Build history of the part. All positions in model axes, mm. Face numbers are marked on the shaded views. A direction names the side the tool comes from. Coordinates: 2 decimals unless noted, no trailing zeros. Order: outer loops, then holes, each group sorted by start corner. A loop starts at its lowest first (then second) coordinate and runs counter-clockwise, first axis right, second up. Notation, with made-up numbers: (84, 47) - (104, 47) arc R10 cw to (104, 60) - close; hole circle Ø4 at (65, 23.25). An arc over 180 degrees is marked (long way). Return JSON: item names as keys, results as strings.
Autodesk Inventor part; units mm, degrees
ref_plane "Work Plane1" through (0, 0, 24) normal (0, 0, 1) x (1, 0, 0)
ref_plane "YZ Plane" through (0, 0, 0) normal (1, 0, 0) x (0, 1, 0)
ref_plane "XZ Plane" through (0, 0, 0) normal (0, 1, 0) x (-1, 0, 0)
sketch "Sketch1" plane through (0, 0, 0) normal (0, 0, 1) x (1, 0, 0)
  line L0 (-9.7719, -3.7131) -> (-29.115, -3.7131)
  line L1 (-29.115, -3.7131) -> (-29.115, -8.7131)
  line L2 (-29.115, -8.7131) -> (-9.115, -8.7131)
  line L3 (-9.115, -8.7131) -> (-9.115, -28.7131)
  line L4 (-9.115, -28.7131) -> (-4.115, -28.7131)
  line L5 (-4.115, -28.7131) -> (-4.115, -9.37)
  line L6 (-9.7719, -3.7131) -> (27.9352, 33.994)
  line L7 (33.5921, 28.3372) -> (-4.115, -9.37)
  circle A0 centre (32.885, 33.2869) radius 1.85
  arc A1 (33.5921, 28.3372) -> (27.9352, 33.994) centre (32.885, 33.2869) ccw
  dimension "d0" = 20
  dimension "d1" = 20
  dimension "d2" = 5
  dimension "d3" = 5
  dimension "d7" = 42
  dimension "d8" = 42
  dimension "d9" = 3.7
  dimension "d18" = 5
  dimension "d19" = 135
  dimension "d67" = 8
extrude "Extrusion1" add sketch "Sketch1" along normal blind 30
ref_plane "Work Plane1" through (0, 0, 24) normal (0, 0, 1) x (1, 0, 0)
sketch "Sketch3" plane through (0, 0, 24) normal (0, 0, 1) x (1, 0, 0)
  circle A0 centre (32.885, 33.2869) radius 1.85
  circle A1 centre (32.885, 33.2869) radius 12.5
  point P0 (0, 0)
  dimension "d13" = 25
extrude "Extrusion3" cut sketch "Sketch3" against normal blind 18
sketch "Sketch5" plane through (0, 0, 0) normal (0, 0, -1) x (-1, 0, 0)
  circle A0 centre (-32.885, 33.2869) radius 1.85
  line L0 (29.115, -8.7131) -> (29.115, -3.7131)
  line L1 (29.115, -3.7131) -> (9.7719, -3.7131)
  line L2 (9.7719, -3.7131) -> (-27.9352, 33.994)
  arc A1 (-27.9352, 33.994) -> (-33.5921, 28.3372) centre (-32.885, 33.2869) ccw
  line L3 (-33.5921, 28.3372) -> (4.115, -9.37)
  line L4 (4.115, -9.37) -> (4.115, -28.7131)
  line L5 (4.115, -28.7131) -> (9.115, -28.7131)
  line L6 (9.115, -28.7131) -> (9.115, -8.7131)
  line L7 (9.115, -8.7131) -> (29.115, -8.7131)
  line L8 (4.115, -9.37) -> (9.7719, -3.7131)
  point P0 (0, 0)
extrude "Extrusion5" add sketch "Sketch5" along normal blind 55
sketch "Sketch8" plane through (-9.115, -28.7131, -55) normal (-1, 0, 0) x (0, 0, 1)
  circle A0 centre (10, 10) radius 2.25
  line L0 (85, 0) -> (0, 0)
  line L1 (0, 0) -> (0, 20)
  circle A1 centre (25, 10) radius 2.25
  point P0 (55, 28.7131)
  dimension "d40" = 4.5
  dimension "d41" = 10
  dimension "d42" = 10
  dimension "d43" = 4.5
  dimension "d44" = 10
  dimension "d45" = 15
sketch "Sketch9" plane through (-29.115, -3.7131, 30) normal (0, 1, 0) x (1, 0, 0)
  circle A0 centre (10, 75) radius 2.25
  circle A1 centre (10, 60) radius 2.25
  line L0 (0, 85) -> (19.3431, 85)
  line L1 (0, 0) -> (0, 85)
  point P0 (29.115, 30)
  dimension "d46" = 10
  dimension "d47" = 10
  dimension "d48" = 10
  dimension "d49" = 15
  dimension "d50" = 4.5
  dimension "d51" = 4.5
extrude "Extrusion8" cut sketch "Sketch9" against normal mid plane 20
extrude "Extrusion9" cut sketch "Sketch8" against normal blind 20
sketch "Sketch10" plane through (0, 0, 30) normal (0, 0, 1) x (1, 0, 0)
  line L0 (-10.9341, 2.1461) -> (2.7686, -11.5566)
  line L1 (2.7686, -11.5566) -> (2.7686, -32.7748)
  line L2 (2.7686, -32.7748) -> (-29.9337, -32.7748)
  line L3 (-29.9337, -32.7748) -> (-29.9337, 2.1461)
  line L4 (-29.9337, 2.1461) -> (-10.9341, 2.1461)
  line L5 (-8.915, -8.5131) -> (-0.2749, -8.5131)
  line L6 (-8.915, -8.5131) -> (-8.915, 0.127)
  line L7 (-9.115, -8.7131) -> (-9.115, -28.7131)
  point P0 (0, 0)
  point P1 (-4.0828, -4.7053)
  dimension "d56" = 135
  dimension "d65" = 0.2
  dimension "d66" = 0.2
extrude "Extrusion10" cut sketch "Sketch10" against normal blind 48 contours L0 L6 L5 L1 L2 L3 L4
sketch "Sketch12" plane through (0, 0, 30) normal (0, 0, 1) x (1, 0, 0)
  line L0 (-8.915, -8.5131) -> (-3.2582, -8.5131)
  line L1 (-3.2582, -8.5131) -> (-8.915, -8.5131)
  line L2 (-8.915, -8.5131) -> (-8.915, 41.4826)
  line L3 (-8.915, 41.4826) -> (-3.915, 41.4826)
  line L4 (-8.915, -2.8562) -> (-8.915, -8.5131)
  line L5 (-8.915, -8.5131) -> (41.085, -8.5131)
  line L6 (41.085, -8.5131) -> (41.085, -3.5131)
  line L7 (41.085, -3.5131) -> (-8.915, -3.5131)
  line L8 (-8.915, -3.5131) -> (-8.915, -8.5131)
  line L9 (-3.915, -8.5131) -> (-3.915, 41.4826)
  point P0 (0, 0)
  point P1 (-8.915, -3.5131)
  point P2 (-3.915, -3.5131)
  dimension "d68" = 5
  dimension "d70" = 50
  dimension "d71" = 50
  dimension "d75" = 0
  dimension "d76" = 5
extrude "Extrusion12" add sketch "Sketch12" against normal blind 20
sketch "Sketch13" plane through (-3.915, 2.1438, 30) normal (1, 0, 0) x (0, 0, -1)
  circle A0 centre (10, 34.3388) radius 2.25
  line L0 (0, 0) -> (0, 39.3388)
  line L1 (0, 39.3388) -> (20, 39.3388)
  point P0 (30, -2.1438)
  dimension "d77" = 10
  dimension "d78" = 5
  dimension "d79" = 4.5
sketch "Sketch14" plane through (1.7418, -3.5131, 30) normal (0, 1, 0) x (1, 0, 0)
  circle A0 centre (34.3431, 10) radius 2.25
  line L0 (39.3431, 0) -> (39.3431, 20)
  line L1 (39.3431, 0) -> (0, 0)
  point P0 (-1.7418, 30)
  dimension "d80" = 5
  dimension "d81" = 4.5
  dimension "d82" = 10
extrude "Extrusion13" cut sketch "Sketch13" against normal blind 20
extrude "Extrusion14" cut sketch "Sketch14" against normal blind 20
sketch "Sketch15" plane through (0, 0, -55) normal (0, 0, -1) x (-1, 0, 0)
  line L0 (-27.9352, 33.994) -> (3.915, 2.1438)
  line L1 (-16.0867, 22.1455) -> (-21.7436, 16.4887)
  line L2 (-1.7418, -3.5131) -> (-33.5921, 28.3372)
  line L3 (-24.5175, 13.7148) -> (-29.4962, 12.412)
  circle A0 centre (-32.885, 33.2869) radius 1.85
  line L4 (29.115, -8.7131) -> (29.115, -3.7131)
  line L5 (29.115, -3.7131) -> (9.7719, -3.7131)
  line L6 (9.7719, -3.7131) -> (-27.9352, 33.994)
  arc A1 (-27.9352, 33.994) -> (-33.5921, 28.3372) centre (-32.885, 33.2869) ccw
  line L7 (-33.5921, 28.3372) -> (4.115, -9.37)
  line L8 (4.115, -9.37) -> (4.115, -28.7131)
  line L9 (4.115, -28.7131) -> (9.115, -28.7131)
  line L10 (9.115, -28.7131) -> (9.115, -8.7131)
  line L11 (9.115, -8.7131) -> (29.115, -8.7131)
  point P0 (0, 0)
extrude "Extrusion15" cut sketch "Sketch15" against normal blind 55 contours L0 L1 L2 A1
equation "\"d8\" = d7"
equation "\"d43\" = d40"
equation "\"d44\" = d41"
equation "\"d71\" = d70"
equation "\"RodDiameter\" = 8"
equation "\"VerticalBearingOD\" = 16"
equation "\"PrintingClearance\" = 0.2"
equation "\"TubeID\" = 18"
equation "\"XLinearBearingOD\" = 19"
properties part number "PulleyHolderXY" material "PET Plastic"
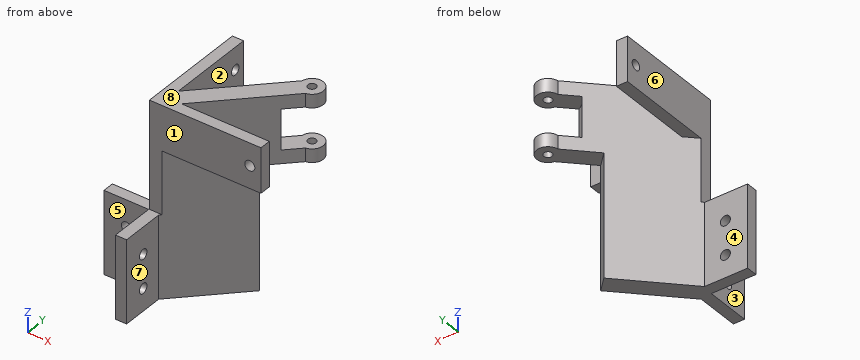
1. Cut at C-C on z = 8. Give the cut face in (x, y) (1 decimal).
Check values:
{"outline": "(-8.9, -8.5) - (-3.3, -8.5) - (27.3, 22.1) arc R12.5 cw to (21.7, 27.7) - (-8.9, -2.9) - close"}
2. Tool access for the marked faces 4, 5, 6, 7 and 8: list every direction of +Z, -Z, +X, -X, +Y, -Y with a clear straight run to the whole face (end or side of a thin tool).
Check values:
{"face 4": "+Z, -Z, -X, +Y", "face 5": "+Z, -Z, -X, -Y", "face 6": "+Z, -X, +Y, -Y", "face 7": "+Z, -Z, +X, -Y", "face 8": "+Z, +X, -X, +Y, -Y"}
3. Cut at A-A on z = -30. Give the cut face in (x, y) (1 decimal).
Check values:
{"outline": "(-29.1, -8.7) - (-21.4, -8.7) - (-21.4, -3.7) - (-29.1, -3.7) - close; (-16.9, -8.7) - (-9.1, -8.7) - (-9.1, -16.5) - (-4.1, -16.5) - (-4.1, -9.4) - (21.7, 16.5) - (16.1, 22.1) - (-9.8, -3.7) - (-16.9, -3.7) - close; (-9.1, -28.7) - (-4.1, -28.7) - (-4.1, -21) - (-9.1, -21) - close"}
4. Cut at B-B on x = 6. Give the cut face in (y, z).
Check values:
{"outline": "(-8.51, 10) - (-3.51, 10) - (-3.51, 30) - (-8.51, 30) - close; (0.75, -55) - (12.06, -55) - (12.06, 30) - (0.75, 30) - close"}
5. Probe L1, parallel to X at y = -5, z = 20 (3 decimals); L2, parallel to Y at x = -7.35, z = 20; L3, parallel to X at y = 9, z = 0.5. List the from-to ranges inside material, lowest first.
Check values:
{"L1": "-8.915 to 33.835, 38.335 to 41.085", "L2": "-8.51 to 34.23, 38.73 to 41.48", "L3": "2.94 to 14.25"}
6. Cut at D-D on y = -7. Give the cut face in (x, z) (3 decimals), plus the area to 3 significant figures.
Check values:
{"outline": "(-29.115, -55) - (-1.745, -55) - (-1.745, 10) - (41.085, 10) - (41.085, 30) - (-8.915, 30) - (-8.915, -18) - (-29.115, -18) - close; hole circle Ø4.5 at (-19.115, -45); hole circle Ø4.5 at (-19.115, -30); hole circle Ø4.5 at (36.085, 20)", "area": "2,170 mm²"}
7. Mould opens along X. For the marked faces 1, 2 and 3 say: pulls with the +X half, pulls with the -X half, needs draft (parallel to the pull), parting line crosses it, or undercut.
Check values:
{"face 1": "needs draft", "face 2": "undercut", "face 3": "pulls with the -X half"}
8. Drop flat-ended pins along their axis: pin 1 (14.5 mm diameter, centred on x = 14.5, z = 4, fed in from -Y); pin 2 (8 mm diameter, centred on x = 30.5, y = -10.5, fed in from -Z); pin 3 (12 mm diameter, centred on x = 18, y = -3, fed in from +Z); pin 4 (6 mm diameter, centred on y = -8, z = -13, fed in from +X) (3 decimals). Give the stop position or say it passes through.
Check values:
{"pin 1": "y = -8.51", "pin 2": "z = 10", "pin 3": "z = 30", "pin 4": "x = 0.255"}
